Autodesk Inventor part; units mm, degrees
ref_plane "YZ Plane" through (0, 0, 0) normal (1, 0, 0) x (0, 1, 0)
ref_plane "XZ Plane" through (0, 0, 0) normal (0, 1, 0) x (-1, 0, 0)
ref_plane "XY Plane" through (0, 0, 0) normal (0, 0, 1) x (1, 0, 0)
sketch "Sketch1" plane through (0, 0, 0) normal (0, 0, 1) x (1, 0, 0)
  circle A0 centre (0, 0) radius 5.1562
  circle A1 centre (0, 0) radius 10.3124
  dimension "d0" = 10.3124
  dimension "d1" = 20.6248
extrude "Extrusion1" add sketch "Sketch1" along normal blind 2.794
fillet "Fillet1" radius 0.254 2 edges at (-10.3124, 0, 2.794) (-10.3124, 0, 0)
fillet "Fillet2" radius 0.254 2 edges at (-5.1562, 0, 2.794) (-5.1562, 0, 0)
properties part number "375 washer structural 112 thick" material "Steel"
For this review, take the finished solid that the model builds, in its own axes (mm). Round coordinates to 2 decimals unless told otherwise and drop trailing zeros. Loops run counter-clockwise (first coordinate to the right, second up) from the corner with the lowest first, then second, coordinate; pieces in that order, holes last. Notation, with made-up numbers: (21.25, 13.5) - (73.25, 13.5) arc R34 ccw to (73.25, 49.5) - close; hole circle Ø11 at (1, 42). An arc over 180 degrees is marked (long way). Use one line per item in the form item = value.
Item 1: Consider section A-A on y = 0. Write out the cut boundary in (x, z), then the cut area to 3 significant figures.
Answers:
outline = (-10.31, 0.25) arc R0.25 ccw to (-10.06, 0) - (-5.41, 0) arc R0.25 ccw to (-5.16, 0.25) - (-5.16, 2.54) arc R0.25 ccw to (-5.41, 2.79) - (-10.06, 2.79) arc R0.25 ccw to (-10.31, 2.54) - close; (5.16, 0.25) arc R0.25 ccw to (5.41, 0) - (10.06, 0) arc R0.25 ccw to (10.31, 0.25) - (10.31, 2.54) arc R0.25 ccw to (10.06, 2.79) - (5.41, 2.79) arc R0.25 ccw to (5.16, 2.54) - close
area = 28.7 mm^2
Item 2: Consider section C-C on z = 1.45. Write out the cut boundary in (x, y).
Answers:
outline = circle Ø20.62 at (0, 0); hole circle Ø10.31 at (0, 0)
Item 3: Clearance check with flat-ended pins moving along their axes: P1, Ø1, axis at x = -6.5, z = 0.5, coming from the -Y side; P2, Ø1, axis at y = -3, z = 0.5, coming from the -X side. State where each tip first meets the part, or that it passes through.
Answers:
P1 = -8.39
P2 = -10
Item 4: Mouldability with a two-part tool opening along X and no side actions: class faces 1 (the cylindrical face through (5.54, -8.7, 1.38)), 2 (the cylindrical face through (2.77, -4.35, 1.38)), 3 (the flat face through (4, -4, 0)) as +X half, -X half, draft (parallel to the pull), parting line (faces both ways), or undercut.
Answers:
face_1 = parting line
face_2 = undercut
face_3 = draft
Item 5: For line 1 (Y direction, x = 0, z = 1.7); line 2 (Y direction, x = -1.5, z = 1.2); line 3 (X direction, y = -1.25, z = 0.75), list the stretches that pass through material, from the lowest coordinate up.
Answers:
line_1 = -10.31 to -5.16, 5.16 to 10.31
line_2 = -10.2 to -4.93, 4.93 to 10.2
line_3 = -10.24 to -5, 5 to 10.24
